Verification items for the finished model (mm, model axes). Round coordinates to 2 decimals unless told otherwise and drop trailing zeros. Order: outer loops, then holes, each group sorted by start corner. A loop starts at its lowest first (then second) coordinate and runs counter-clockwise, first axis right, second up. Notation, with made-up numbers: (61, 54) -> (118, 54) arc R18 ccw to (118, 70) -> close; hole circle Ø4 at (43.5, 84.25). An arc over 180 degrees is marked (long way). Put each result on its own line as item: value.
```python
from build123d import *

# Parameters (mm, degrees)
ESQUISSE1_W             = 50
ESQUISSE1_H             = 70
ESQUISSE1_R             = 5
ESQUISSE1_R_2           = 5.055
ESQUISSE1_R_3           = 2.065
BASE_EXTRUSION_DEPTH    = 15
CHANFREIN3_SIZE         = 5
ENL_V_MAT_EXTRU_1_REACH = 77.829
ESQUISSE2_R             = 2.065


with BuildPart() as part:
    # Esquisse1 → Base-Extrusion (new body)
    with BuildSketch(Plane.XY):
        with Locations((0, 35)):
            Rectangle(ESQUISSE1_W, ESQUISSE1_H)
        with Locations((15, 13)):
            Circle(ESQUISSE1_R, mode=Mode.SUBTRACT)
        with Locations(Location((-15, 13, 0), (0, 0, 180))):
            Circle(ESQUISSE1_R, mode=Mode.SUBTRACT)
        with Locations((0, 35)):
            Circle(ESQUISSE1_R_2, mode=Mode.SUBTRACT)
        with Locations((-15, 60)):
            Circle(ESQUISSE1_R_3, mode=Mode.SUBTRACT)
        with Locations(Location((15, 60, 0), (0, 0, 180))):
            Circle(ESQUISSE1_R_3, mode=Mode.SUBTRACT)
    extrude(amount=BASE_EXTRUSION_DEPTH)

    # Chanfrein3
    chanfrein3_edges = [part.edges().sort_by_distance(p)[0] for p in [
        (0, 70, 0),
    ]]
    chamfer(chanfrein3_edges, length=CHANFREIN3_SIZE)

    # Esquisse2 → Enlèv. mat.-Extru.1 (cut, up to next)
    with BuildSketch(Plane.XZ, mode=Mode.PRIVATE) as enl_v_mat_extru_1_sk1:
        with Locations(Location((15, 7.5, 0), (0, 0, 270))):
            Circle(ESQUISSE2_R)
    enl_v_mat_extru_1_tool1 = extrude(enl_v_mat_extru_1_sk1.sketch, amount=-ENL_V_MAT_EXTRU_1_REACH, mode=Mode.PRIVATE) & part.part
    # Esquisse2 → Enlèv. mat.-Extru.1 (cut, up to next)
    with BuildSketch(Plane.XZ, mode=Mode.PRIVATE) as enl_v_mat_extru_1_sk2:
        with Locations(Location((-15, 7.5, 0), (0, 0, 270))):
            Circle(ESQUISSE2_R)
    enl_v_mat_extru_1_tool2 = extrude(enl_v_mat_extru_1_sk2.sketch, amount=-ENL_V_MAT_EXTRU_1_REACH, mode=Mode.PRIVATE) & part.part
    add(enl_v_mat_extru_1_tool1.solids().sort_by_distance((15, 0, 7.5))[0], mode=Mode.SUBTRACT)
    add(enl_v_mat_extru_1_tool2.solids().sort_by_distance((-15, 0, 7.5))[0], mode=Mode.SUBTRACT)


solid = part.part
```
Item 1: Sectioned sample at A-A, the plane y = 35. Record the boundary of the cut face in (x, z) (3 decimals), then the cut area to 3 significant figures.
Geometry check:
outline: (-25, 0) -> (-5.055, 0) -> (-5.055, 15) -> (-25, 15) -> close; (5.055, 0) -> (25, 0) -> (25, 15) -> (5.055, 15) -> close
area: 598 mm2
Item 2: Depth check by flat-ended pin: pin 1 Ø3.5 at (x, y) = (-15, 60) entering from -Z. Enter the tip coordinate at first touch or a pass-through.
Geometry check:
pin 1: through
Item 3: Sectioned sample at D-D, the plane z = 1.75. Record the boundary of the cut face in (x, y) (3 decimals).
Geometry check:
outline: (-25, 0) -> (25, 0) -> (25, 66.75) -> (-25, 66.75) -> close; hole circle Ø10 at (-15, 13); hole circle Ø4.13 at (-15, 60); hole circle Ø10.11 at (0, 35); hole circle Ø10 at (15, 13); hole circle Ø4.13 at (15, 60)
Item 4: Sectioned sample at B-B, the plane x = 0. Record the boundary of the cut face in (y, z) (3 decimals), then the cut area to 3 significant figures.
Geometry check:
outline: (0, 0) -> (29.945, 0) -> (29.945, 15) -> (0, 15) -> close; (40.055, 0) -> (65, 0) -> (70, 5) -> (70, 15) -> (40.055, 15) -> close
area: 886 mm2
Item 5: Material ranges on line 1 along Y through (x, z) = (15, 10.25) (3 decimals); line 2 along Z through (x, y) = (-15, 4) (3 decimals); line 3 along Y through (x, z) = (-15, 8.5) (3 decimals), recorded low to high.
Geometry check:
line 1: 0 to 8, 18 to 57.935, 62.065 to 70
line 2: 0 to 5.435, 9.565 to 15
line 3: 18 to 57.935, 62.065 to 70
Item 6: Sectioned sample at C-C, the plane x = -15. Record the boundary of the cut face in (y, z) (3 decimals), then the cut area to 3 significant figures.
Geometry check:
outline: (0, 0) -> (8, 0) -> (8, 5.435) -> (0, 5.435) -> close; (0, 9.565) -> (8, 9.565) -> (8, 15) -> (0, 15) -> close; (18, 0) -> (57.935, 0) -> (57.935, 15) -> (18, 15) -> close; (62.065, 0) -> (65, 0) -> (70, 5) -> (70, 15) -> (62.065, 15) -> close
area: 793 mm2
Item 7: Release check for a two-part mould opening along Z. For faces 1 (the face through (-6, 33, 0)), 2 (the face through (-12.953, 4.164, 7.769)), 3 (the face through (17.047, 4.164, 7.769)), 4 (the face through (0, 0, 7)) record: pulls with the +Z half, pulls with the -Z half, needs draft (parallel to the pull), parting line crosses it, or undercut.
Geometry check:
face 1: pulls with the -Z half
face 2: undercut
face 3: undercut
face 4: needs draft
